Job drawing, mm, ordinate dimensions from the low corner. One solid piece. Coordinates: 2 decimals unless noted, no trailing zeros. Order: outer loops, then holes, each group sorted by start corner. A loop starts at its lowest first (then second) coordinate and runs counter-clockwise, first axis right, second up. Notation, with made-up numbers: (-27.75, 72.25) - (22.25, 72.25) arc R18 cw to (22.25, 80.25) - close; hole circle Ø2 at (-11, -35). An arc over 180 degrees is marked (long way). Use one line per item in the form item = value.
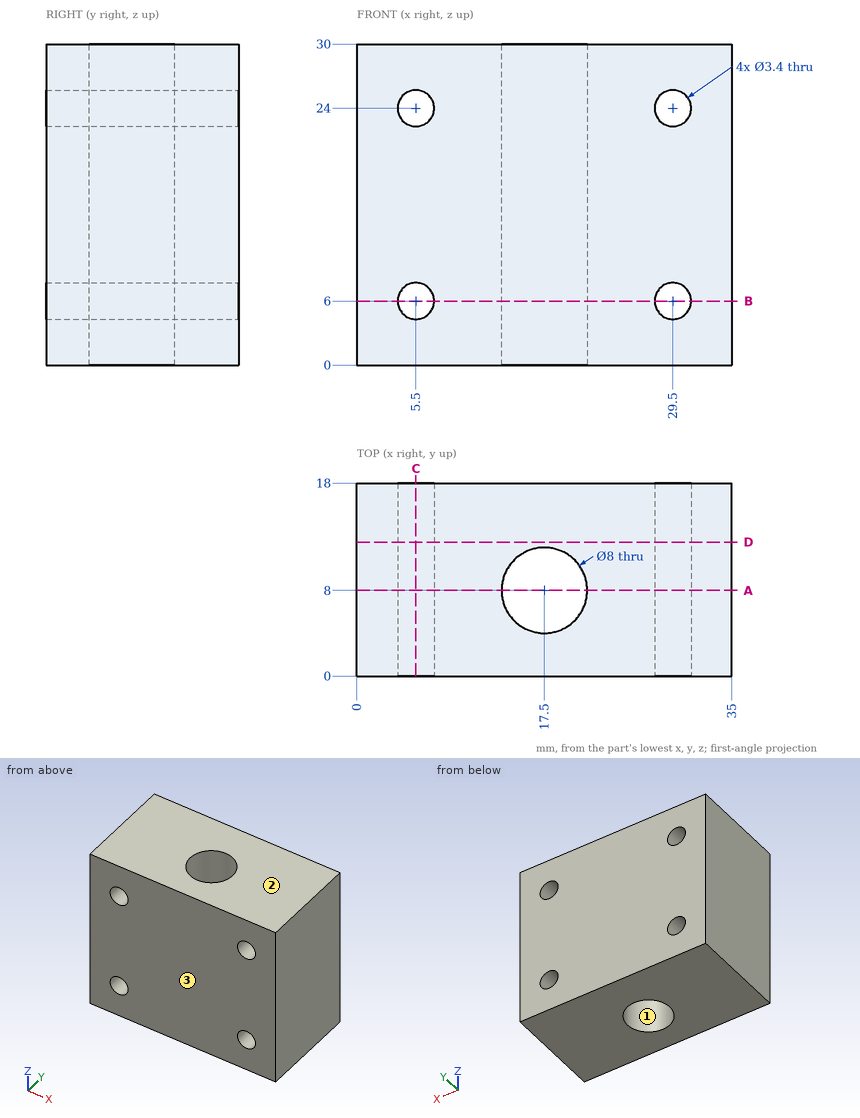
Item 1: Drop a flat-ended pin along its axis: pin 1 (6.5 mm diameter, centred on x = 17.5, y = 8, fed in from +Z). Give the stop position or say it passes through.
Derived:
pin_1 = through
Item 2: Drill centre lines: line 1 (Y direction, x = 17.5, z = 21.5); line 2 (X direction, y = 13.5, z = 24); line 3 (X direction, y = 9.75, z = 6). Where is each one in solid material? Low to high. Write a range as [from, to].
Derived:
line_1 = [0, 4], [12, 18]
line_2 = [0, 3.8], [7.2, 27.8], [31.2, 35]
line_3 = [0, 3.8], [7.2, 13.9], [21.1, 27.8], [31.2, 35]
Item 3: Cut at D-D, the plane y = 12.5. Write the cut outline in (x, z).
Derived:
outline = (0, 0) - (35, 0) - (35, 30) - (0, 30) - close; hole circle Ø3.4 at (5.5, 6); hole circle Ø3.4 at (5.5, 24); hole circle Ø3.4 at (29.5, 6); hole circle Ø3.4 at (29.5, 24)
Item 4: Cut at B-B, the plane z = 6. Write the cut outline in (x, y), plus the area to 3 significant figures.
Derived:
outline = (0, 0) - (3.8, 0) - (3.8, 18) - (0, 18) - close; (7.2, 0) - (27.8, 0) - (27.8, 18) - (7.2, 18) - close; (31.2, 0) - (35, 0) - (35, 18) - (31.2, 18) - close; hole circle Ø8 at (17.5, 8)
area = 457 mm²
Item 5: Cut at C-C, the plane x = 5.5. Write the cut outline in (y, z).
Derived:
outline = (0, 0) - (18, 0) - (18, 4.3) - (0, 4.3) - close; (0, 7.7) - (18, 7.7) - (18, 22.3) - (0, 22.3) - close; (0, 25.7) - (18, 25.7) - (18, 30) - (0, 30) - close
Item 6: Two-plate mould, pull along Y, no slides. Class the marked faces 1, 2 and 3: +Y half, -Y half, draft (parallel to the pull), parting line (faces both ways), or undercut.
Derived:
face_1 = undercut
face_2 = draft
face_3 = -Y half
Item 7: Cut at A-A, the plane y = 8. Write the cut outline in (x, z).
Derived:
outline = (0, 0) - (13.5, 0) - (13.5, 30) - (0, 30) - close; (21.5, 0) - (35, 0) - (35, 30) - (21.5, 30) - close; hole circle Ø3.4 at (5.5, 6); hole circle Ø3.4 at (5.5, 24); hole circle Ø3.4 at (29.5, 6); hole circle Ø3.4 at (29.5, 24)
